The listing builds one solid part. Answer for the finished solid, in the listing's coordinates (mm). Face numbers are marked on the shaded views. A direction names the side the tool comes from. Give positions to 0.01 mm unless a question says otherwise; leave off trailing zeros. Loops run counter-clockwise (first coordinate to the right, second up) from the corner with the lowest first, then second, coordinate; pieces in that order, holes last. Notation, with made-up numbers: (-15, 0) - (-1, 0) arc R16 ccw to (-1, 15) - close; hole circle Ø5 at (-35.75, 29.5). An arc over 180 degrees is marked (long way). Write each question's results on one line, items separated by ' | '.
from build123d import *

# Parameters (mm, degrees)
SKETCH_1_W          = 20
SKETCH_1_H          = 20
EXTRUDE_1_DEPTH     = 3
SKETCH_2_W          = 7
SKETCH_2_H          = 6
EXTRUDE_2_DEPTH     = 40
SKETCH_3_W          = 3
SKETCH_3_H          = 20
EXTRUDE_3_DEPTH     = 25
CUT_EXTRUDE_1_REACH = 49.212
SKETCH_4_R          = 2.6
FILLET_1_R          = 1
SKETCH_5_W          = 3.2
SKETCH_5_H          = 3.9
CUT_EXTRUDE_2_DEPTH = 30
SKETCH_6_W          = 6
SKETCH_6_H          = 9.5
EXTRUDE_4_DEPTH     = 43
CHAMFER_1_SIZE      = 0.5
SKETCH_7_W          = 6.4
SKETCH_7_H          = 9.5
EXTRUDE_5_DEPTH     = 16.5
EXTRUDE_6_DEPTH     = 25
FILLET_2_R          = 2
EXTRUDE_7_DEPTH     = 43
SKETCH_10_W         = 1.9
SKETCH_10_H         = 2
CUT_EXTRUDE_3_DEPTH = 26.5
FILLET_3_R          = 0.5
FILLET_4_R          = 1.5


with BuildPart() as part:
    # ｽｹｯﾁ1 → ﾎﾞｽ - 押し出し1 (new body)
    with BuildSketch(Plane.XY):
        Rectangle(SKETCH_1_W, SKETCH_1_H)
    extrude(amount=EXTRUDE_1_DEPTH)

    # ｽｹｯﾁ2 → ﾎﾞｽ - 押し出し2 (add)
    with BuildSketch(Plane(origin=(0, 0, 0), x_dir=(-1, 0, 0), z_dir=(0, 0, -1))):
        with Locations((0, 7)):
            Rectangle(SKETCH_2_W, SKETCH_2_H)
    extrude(amount=EXTRUDE_2_DEPTH)

    # ｽｹｯﾁ3 → ﾎﾞｽ - 押し出し3 (add)
    with BuildSketch(Plane.XY.offset(3)):
        with Locations((11.5, 0)):
            Rectangle(SKETCH_3_W, SKETCH_3_H)
    extrude(amount=-EXTRUDE_3_DEPTH)

    # ｽｹｯﾁ4 → ｶｯﾄ - 押し出し1 (cut, up to next)
    with BuildSketch(Plane(origin=(13, 0, 0), x_dir=(0, 0, -1), z_dir=(1, 0, 0)), mode=Mode.PRIVATE) as cut_extrude_1_sk1:
        with Locations(Location((10, 0, 0), (0, 0, 90))):
            Circle(SKETCH_4_R)
    cut_extrude_1_tool1 = extrude(cut_extrude_1_sk1.sketch, amount=-CUT_EXTRUDE_1_REACH, mode=Mode.PRIVATE) & part.part
    add(cut_extrude_1_tool1.solids().sort_by_distance((13, 0, -10))[0], mode=Mode.SUBTRACT)

    # ﾌｨﾚｯﾄ1
    fillet_1_edges = [part.edges().sort_by_distance(p)[0] for p in [
        (-10, -10, 1.5),
    ]]
    fillet(fillet_1_edges, radius=FILLET_1_R)

    # ｽｹｯﾁ5 → ｶｯﾄ - 押し出し2 (cut)
    with BuildSketch(Plane(origin=(0, 0, -13.5), x_dir=(-1, 0, 0), z_dir=(0, 0, -1))):
        with Locations((0, 8.05)):
            Rectangle(SKETCH_5_W, SKETCH_5_H)
    extrude(amount=CUT_EXTRUDE_2_DEPTH, mode=Mode.SUBTRACT)

    # ｽｹｯﾁ6 → ﾎﾞｽ - 押し出し4 (add)
    with BuildSketch(Plane.XY.offset(3)):
        with Locations((6.2, 14.75)):
            Rectangle(SKETCH_6_W, SKETCH_6_H)
        with Locations((-6.2, 14.75)):
            Rectangle(SKETCH_6_W, SKETCH_6_H)
    extrude(amount=-EXTRUDE_4_DEPTH)

    # 面取り1
    chamfer_1_edges = [part.edges().sort_by_distance(p)[0] for p in [
        (-3.5, 10, -20),
        (3.5, 10, -20),
    ]]
    chamfer(chamfer_1_edges, length=CHAMFER_1_SIZE)

    # ｽｹｯﾁ7 → ﾎﾞｽ - 押し出し5 (add)
    with BuildSketch(Plane.XY.offset(3)):
        with Locations((0, 14.75)):
            Rectangle(SKETCH_7_W, SKETCH_7_H)
    extrude(amount=-EXTRUDE_5_DEPTH)

    # ｽｹｯﾁ8 → ﾎﾞｽ - 押し出し6 (add)
    with BuildSketch(Plane.XY.offset(3)):
        Polygon((13, 10), (9.2, 16.581793069), (9.2, 10), align=None)
    extrude(amount=-EXTRUDE_6_DEPTH)

    # ﾌｨﾚｯﾄ2
    fillet_2_edges = [part.edges().sort_by_distance(p)[0] for p in [
        (9.2, 16.581793069, -9.5),
        (13, 10, -9.5),
        (13, -10, -9.5),
        (9.2, 19.5, -18.5),
        (-9.2, 19.5, -18.5),
    ]]
    fillet(fillet_2_edges, radius=FILLET_2_R)

    # ｽｹｯﾁ9 → ﾎﾞｽ - 押し出し7 (add)
    with BuildSketch(Plane.XY.offset(3)):
        Polygon((-10, 10), (-9.2, 15.8), (-9.2, 10), align=None)
    extrude(amount=-EXTRUDE_7_DEPTH)

    # ｽｹｯﾁ10 → ｶｯﾄ - 押し出し3 (cut)
    with BuildSketch(Plane(origin=(0, 0, -40), x_dir=(-1, 0, 0), z_dir=(0, 0, -1))):
        with Locations((2.55, 7.1)):
            Rectangle(SKETCH_10_W, SKETCH_10_H)
    extrude(amount=-CUT_EXTRUDE_3_DEPTH, mode=Mode.SUBTRACT)

    # ﾌｨﾚｯﾄ3
    fillet_3_edges = [part.edges().sort_by_distance(p)[0] for p in [
        (-3.5, 6.1, -26.75),
        (-3.5, 8.1, -26.75),
    ]]
    fillet(fillet_3_edges, radius=FILLET_3_R)

    # ﾌｨﾚｯﾄ4
    fillet_4_edges = [part.edges().sort_by_distance(p)[0] for p in [
        (-3.5, 4, -20),
        (3.5, 4, -20),
    ]]
    fillet(fillet_4_edges, radius=FILLET_4_R)


solid = part.part
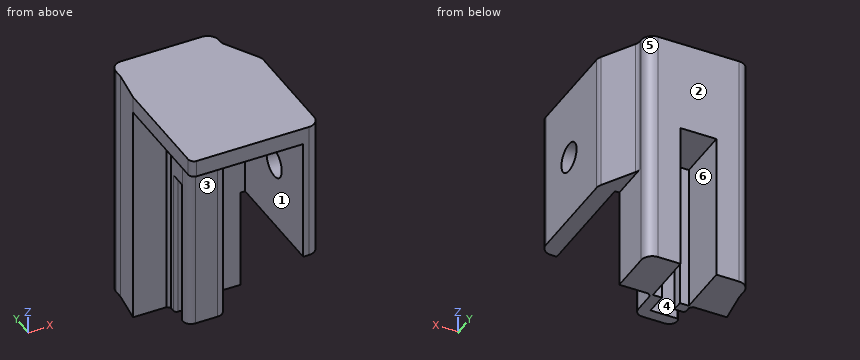
Item 1: For a pull along X with two mould halves and no side action, classify the marked faces 4, 5 and 6 as released by +X, released by -X, zero draft, split by the parting line, or undercut.
Values found:
face 4: zero draft | face 5: released by +X | face 6: undercut
Item 2: A cutting plane is placed at C-C, the plane y = -4.75. Determine the outline of the cut face in (x, z).
Values found:
outline: (-10, 0) - (10, 0) - (10, -22) - (13, -22) - (13, 3) - (-10, 3) - close
Item 3: Flat-ended cylindrical pins translate along their axes: P1, Ø1.3, axis at x = 2.5, z = -21, coming from the +Y side; P2, Ø3, axis at x = 6.5, z = -10, coming from the -Y side; P3, Ø1.5, axis at x = 1.5, y = 14, coming from the -Z side. Find the tip coordinate at first contact, or state that the pin passes through.
Values found:
P1: stops at y = 10 | P2: stops at y = 10 | P3: stops at z = -13.5
Item 4: For the marked faces 1, 2 and 3, determine the directions among +Z, -Z, +X, -X, +Y, -Y from which every point of the face is accessible in a straight line to the end or side of a thin tool.
Values found:
face 1: -Z, -Y | face 2: +Z, -Z, +X, -X, +Y | face 3: -Z, -X, -Y
Item 5: A cutting plane is placed at D-D, the plane z = -10. Determine the outline of the cut face in (x, y).
Values found:
outline: (-10, 10) - (-4, 10) - (-3.5, 9.5) - (-3.5, 5.5) arc R1.5 ccw to (-2, 4) - (2, 4) arc R1.5 ccw to (3.5, 5.5) - (3.5, 9.5) - (4, 10) - (10, 10) - (10, 2.6) - (13, 2.6) - (13, 9.46) arc R2 ccw to (12.73, 10.46) - (9.47, 16.12) arc R2 cw to (9.2, 17.12) - (9.2, 17.5) arc R2 ccw to (7.2, 19.5) - (-7.2, 19.5) arc R2 ccw to (-9.2, 17.5) - (-9.2, 15.8) - close; (10, -10) - (11, -10) arc R2 ccw to (13, -8) - (13, -2.6) - (10, -2.6) - close
Item 6: A cutting plane is placed at B-B, the plane y = 0. Determine the outline of the cut face in (x, z).
Values found:
outline: (-10, 0) - (10, 0) - (10, -7.4) - (13, -7.4) - (13, 3) - (-10, 3) - close; (10, -22) - (13, -22) - (13, -12.6) - (10, -12.6) - close
Item 7: Find the intervals of material crossed by line 1 along X through (y, z) = (16.75, -33.5); line 2 along X through (y, z) = (8.5, -31.5); line 3 along Z through (x, y) = (12.3, 0), in increasing order. Write a range as [from, to].
Values found:
line 1: x = [-9.2, -3.2], [3.2, 9.2] | line 2: x = [-3.49, -1.6], [1.6, 3.5] | line 3: z = [-22, -12.6], [-7.4, 3]
